```python
from build123d import *

# Parameters (mm, degrees)
BOSS_EXTRUDE1_DEPTH      = 50
BOSS_EXTRUDE1_DEPTH_BACK = 50
SKETCH1_W                = 150
SKETCH1_H                = 15
BOSS_EXTRUDE2_DEPTH      = 7.5
BOSS_EXTRUDE2_DEPTH_BACK = 7.5
HOLE1_D                  = 20
BOSS_EXTRUDE3_DEPTH      = 3.75
HOLE2_D                  = 20


with BuildPart() as part:
    # Sketch1 → Boss-Extrude1 (new, two sides: drawn at the far end of the back side and taken through both)
    with BuildSketch(Plane.XY.offset(-BOSS_EXTRUDE1_DEPTH_BACK)):
        with Locations((0, 7.5)):
            Rectangle(SKETCH1_W, SKETCH1_H)
    extrude(amount=BOSS_EXTRUDE1_DEPTH + BOSS_EXTRUDE1_DEPTH_BACK)

    # Sketch2 → Boss-Extrude2 (add, two sides: drawn at the far end of the back side and taken through both)
    with BuildSketch(Plane.XY.offset(-BOSS_EXTRUDE2_DEPTH_BACK)):
        with BuildLine():
            Line((75, 15), (-122.10432852, 99.958128973))
            ThreePointArc((-122.10432852, 99.958128973), (-154.328840447, 88.243793145), (-144.552094943, 55.379525617))
            Line((-144.552094943, 55.379525617), (-75, 15))
            Line((-75, 15), (75, 15))
        make_face()
    extrude(amount=BOSS_EXTRUDE2_DEPTH + BOSS_EXTRUDE2_DEPTH_BACK)

    # Hole1 (through all)
    with Locations(Plane.XY.offset(7.5)):
        with Locations((-132, 77)):
            Hole(HOLE1_D / 2)

    # Sketch5 → Boss-Extrude3 (add, symmetric)
    with BuildSketch(Plane(origin=(0, 0, 0), x_dir=(0, 0, -1), z_dir=(1, 0, 0))):
        Polygon((-50, 15), (-7.5, 35), (-7.5, 15), align=None)
    boss_extrude3 = extrude(amount=BOSS_EXTRUDE3_DEPTH, both=True)

    # Mirror1: Boss-Extrude3 across plane
    add(boss_extrude3.mirror(Plane.XY))

    # Hole2 (through all)
    with Locations(Plane(origin=(0, 15, 0), x_dir=(1, 0, 0), z_dir=(0, 1, 0))):
        with Locations((45, -30), (-45, -30)):
            hole2 = Hole(HOLE2_D / 2)

    # Mirror2: Hole2 across plane
    add(hole2.mirror(Plane.XY), mode=Mode.SUBTRACT)


solid = part.part
```
Could you check a few things on this model? Use its own coordinates, in mm. A direction names the side the tool comes from. Coordinates: 2 decimals unless noted, no trailing zeros. Write each loop counter-clockwise with the first axis right and the second up, starting at its lowest first coordinate (ties: lowest second). Pieces come first, ordered by that corner, then holes. Notation, with made-up numbers: M 28,-5 L 60,-5 A10 ccw 60,5 Z; hole C 46,34 d10. An arc over 180 degrees is marked long. Answer as CSV lines item,"result". Start each with the question number.
1) For P1, Ø16, axis at y = 22, z = -25, coming from the -X side; P2, Ø13, axis at x = -47.5, z = 25.5, coming from the +Y side; P3, Ø3, axis at x = -83, y = 50, coming from the -Z side, each with a flat end and sliding along its axis, tell me the tip position at first contact or that it passes through.
2) For faces 1 (the flat face through (31, 15, -29)), 2 (the flat face through (-3.75, 21, -19)), 3 (the flat face through (-32, 15, 28)), 4 (the flat face through (3.75, 21, 19)), which set-ups out of +Z, -Z, +X, -X, +Y, -Y let a thin tool reach every point of the face, with its end or its side?
3) Please list where these lines run through material, in increasing order: line 1 (Z direction, x = -45, y = 8.25); line 2 (X direction, y = 8.25, z = -30); line 3 (Z direction, x = -35, y = 24.5). Write a range as from..to.
4) I want a section at B-B, the plane z = -35. Please give me the cut outline in (x, y).
5) We'd pull the mould along Z, two halves only. Please class faces 5 (the cylindrical face through (53, 7, 36)), 6 (the flat face through (-32, 15, -29)), 7 (the flat face through (-68, 49, -7.5)): +Z half, -Z half, draft (parallel to the pull), parting line (faces both ways), or undercut.
6) I want a section at A-A, the plane x = 45. Please give me the cut outline in (y, z), and give its area (3 significant figures).
7) I want a section at D-D, the plane x = -139.5. Please give me the cut outline in (y, z).
8) I want a section at C-C, the plane y = 77. Please give me the cut outline in (x, z), and give its area (3 significant figures).
Data:
1,P1,"stops at x = -75"
1,P2,"stops at y = 15"
1,P3,"stops at z = -7.5"
2,face 1,"-Z, +X, +Y"
2,face 2,"-Z, -X, +Y"
2,face 3,"+Z, -X, +Y"
2,face 4,"+Z, +X, +Y"
3,line 1,"z = -50..-40, -20..20, 40..50"
3,line 2,"x = -75..-55, -35..35, 55..75"
3,line 3,"z = -7.5..7.5"
4,outline,"M -75,0 L -53.66,0 L -53.66,15 L -75,15 Z; M -36.34,0 L 36.34,0 L 36.34,15 L 3.75,15 L 3.75,22.06 L -3.75,22.06 L -3.75,15 L -36.34,15 Z; M 53.66,0 L 75,0 L 75,15 L 53.66,15 Z"
5,face 5,"undercut"
5,face 6,"draft"
5,face 7,"-Z half"
6,outline,"M 0,-50 L 15,-50 L 15,-40 L 0,-40 Z; M 0,-20 L 15,-20 L 15,-7.5 L 27.93,-7.5 L 27.93,7.5 L 15,7.5 L 15,20 L 0,20 Z; M 0,40 L 15,40 L 15,50 L 0,50 Z"
6,area,"1,090 mm^2"
7,outline,"M 52.45,-7.5 L 70.39,-7.5 L 70.39,7.5 L 52.45,7.5 Z; M 83.61,-7.5 L 100.85,-7.5 L 100.85,7.5 L 83.61,7.5 Z"
8,outline,"M -157,-7.5 L -142,-7.5 L -142,7.5 L -157,7.5 Z; M -122,-7.5 L -68.84,-7.5 L -68.84,7.5 L -122,7.5 Z"
8,area,"1,020 mm^2"
